Geometry check sheet. Reference: the model listing, model coordinates, mm. A direction names the side the tool comes from. Coordinates: 2 decimals unless noted, no trailing zeros. Order: outer loops, then holes, each group sorted by start corner. A loop starts at its lowest first (then second) coordinate and runs counter-clockwise, first axis right, second up. Notation, with made-up numbers: (36.5, 8.5) - (79.5, 8.5) arc R6 ccw to (79.5, 17.5) - close; hole circle Ø6 at (16.5, 34). An arc over 180 degrees is marked (long way). Return JSON: item names as keys, results as strings. Group by question number.
Item 1: Gauge pin test, flat ends, axial feed: pin 1 (7 mm diameter, centred on x = 54.9, z = 32.5, fed in from -Y); pin 2 (4.5 mm diameter, centred on x = 54.9, z = 92.5, fed in from +Y); pin 3 (8 mm diameter, centred on x = 40.5, y = 24, fed in from -Z). Record the tip position at first contact, or that the pin passes through.
Item 2: Section check B-B on x = 19.9. Enter the section's corners in (y, z), then the cut area to 3 significant figures.
Item 3: Section check A-A on y = 24.9. Enter the section's corners in (x, z), then the cut area to 3 significant figures.
Item 4: Section check D-D on z = 53. Enter the section's corners in (x, y), then the cut area to 3 significant figures.
Item 5: Tool access check on faces 4 (the cylindrical face through (26.908, 28.204, 7.395)), 5 (the cylindrical face through (43.394, 25.164, 69.23)), 6 (the cylindrical face through (60.85, 4.93, 93.28)). Record the directions out of +Z, -Z, +X, -X, +Y, -Y that give a thin tool (end or side, any length) a straight path to the whole face; none if there is none.
Item 6: Scan lines: probe 1 along Z at (x, y) = (54.9, 38); probe 2 along X at (y, z) = (4.25, 92.5); probe 3 along Y at (x, z) = (37.4, 85). Record each from-to range of solid material in increasing order.
Item 7: Draft check along Z on faces 1 (the flat face through (33, 20, 15)), 2 (the flat face through (0, 25, 62)), 3 (the flat face through (52, 10, 31)). Enter one of: pulls with the +Z half, pulls with the -Z half, needs draft (parallel to the pull), parting line crosses it, or undercut.
Item 8: Section check C-C on z = 32.5. Enter the section's corners in (x, y).
from build123d import *

# Parameters (mm, degrees)
SKETCH1_W                        = 74.8
SKETCH1_H                        = 49.8
SLIDER_BODY_DEPTH                = 125
SKETCH2_R                        = 11
LEAD_NUT_INSET_DEPTH             = 15
SKETCH3_R                        = 6
LEADSCREW_CLEARANCE_DEPTH        = 143.039008726
CORNER_BREAK_R                   = 0.5
BOLT_CLEARANCE_HOLES_D           = 5.5
SKETCH7_R                        = 6
NUT_CLEARANCE_COUNTERBORES_DEPTH = 10


with BuildPart() as part:
    # Sketch1 → slider body (new body)
    with BuildSketch(Plane.XY):
        with Locations((37.4, 24.9)):
            Rectangle(SKETCH1_W, SKETCH1_H)
    extrude(amount=SLIDER_BODY_DEPTH)

    # Sketch2 → lead nut inset (cut)
    with BuildSketch(Plane(origin=(0, 0, 0), x_dir=(-1, 0, 0), z_dir=(0, 0, -1))):
        with Locations((-37.4, 24.9)):
            Circle(SKETCH2_R)
    extrude(amount=-LEAD_NUT_INSET_DEPTH, mode=Mode.SUBTRACT)

    # Sketch3 → leadscrew clearance (cut, through all)
    with BuildSketch(Plane(origin=(0, 0, 15), x_dir=(-1, 0, 0), z_dir=(0, 0, -1))):
        with Locations((-37.4, 24.9)):
            Circle(SKETCH3_R)
    extrude(amount=-LEADSCREW_CLEARANCE_DEPTH, mode=Mode.SUBTRACT)

    # corner break
    corner_break_edges = [part.edges().sort_by_distance(p)[0] for p in [
        (74.8, 24.9, 125),
        (37.4, 49.8, 125),
        (0, 24.9, 125),
        (37.4, 49.8, 0),
        (74.8, 24.9, 0),
        (37.4, 0, 0),
        (0, 24.9, 0),
        (37.4, 0, 125),
        (0, 49.8, 62.5),
        (74.8, 49.8, 62.5),
        (74.8, 0, 62.5),
        (0, 0, 62.5),
    ]]
    fillet(corner_break_edges, radius=CORNER_BREAK_R)

    # bolt clearance holes (through all)
    with Locations(Plane(origin=(0, 49.8, 0), x_dir=(1, 0, 0), z_dir=(0, 1, 0))):
        with Locations((54.9, -92.5), (19.9, -32.5), (54.9, -32.5), (19.9, -92.5)):
            Hole(BOLT_CLEARANCE_HOLES_D / 2)

    # Sketch7 → nut clearance counterbores (cut)
    with BuildSketch(Plane.XZ):
        with Locations(Location((19.9, 92.5, 0), (0, 0, 270))):
            Circle(SKETCH7_R)
        with Locations(Location((54.9, 92.5, 0), (0, 0, 270))):
            Circle(SKETCH7_R)
        with Locations(Location((54.9, 32.5, 0), (0, 0, 270))):
            Circle(SKETCH7_R)
        with Locations(Location((19.9, 32.5, 0), (0, 0, 270))):
            Circle(SKETCH7_R)
    extrude(amount=-NUT_CLEARANCE_COUNTERBORES_DEPTH, mode=Mode.SUBTRACT)


solid = part.part
Computed:
{
 "1": {"pin 1": "stops at y = 10", "pin 2": "passes through", "pin 3": "stops at z = 15"},
 "2": {"outline": "(0, 0.5) arc R0.5 ccw to (0.5, 0) - (49.3, 0) arc R0.5 ccw to (49.8, 0.5) - (49.8, 29.75) - (10, 29.75) - (10, 26.5) - (0, 26.5) - close; (0, 38.5) - (10, 38.5) - (10, 35.25) - (49.8, 35.25) - (49.8, 89.75) - (10, 89.75) - (10, 86.5) - (0, 86.5) - close; (0, 98.5) - (10, 98.5) - (10, 95.25) - (49.8, 95.25) - (49.8, 124.5) arc R0.5 ccw to (49.3, 125) - (0.5, 125) arc R0.5 ccw to (0, 124.5) - close", "area": "5,550 mm²"},
 "3": {"outline": "(0, 0.5) arc R0.5 ccw to (0.5, 0) - (26.4, 0) - (26.4, 15) - (31.4, 15) - (31.4, 125) - (0.5, 125) arc R0.5 ccw to (0, 124.5) - close; (43.4, 15) - (48.4, 15) - (48.4, 0) - (74.3, 0) arc R0.5 ccw to (74.8, 0.5) - (74.8, 124.5) arc R0.5 ccw to (74.3, 125) - (43.4, 125) - close; hole circle Ø5.5 at (19.9, 32.5); hole circle Ø5.5 at (19.9, 92.5); hole circle Ø5.5 at (54.9, 32.5); hole circle Ø5.5 at (54.9, 92.5)", "area": "7,600 mm²"},
 "4": {"outline": "(0, 0.5) arc R0.5 ccw to (0.5, 0) - (74.3, 0) arc R0.5 ccw to (74.8, 0.5) - (74.8, 49.3) arc R0.5 ccw to (74.3, 49.8) - (0.5, 49.8) arc R0.5 ccw to (0, 49.3) - close; hole circle Ø12 at (37.4, 24.9)", "area": "3,610 mm²"},
 "5": {"face 4": "-Z", "face 5": "+Z, -Z", "face 6": "-Y"},
 "6": {"probe 1": "z = 0 to 29.75, 35.25 to 89.75, 95.25 to 125", "probe 2": "x = 0 to 13.9, 25.9 to 48.9, 60.9 to 74.8", "probe 3": "y = 0 to 18.9, 30.9 to 49.8"},
 "7": {"face 1": "pulls with the -Z half", "face 2": "needs draft", "face 3": "undercut"},
 "8": {"outline": "(0, 0.5) arc R0.5 ccw to (0.5, 0) - (13.9, 0) - (13.9, 10) - (17.15, 10) - (17.15, 49.8) - (0.5, 49.8) arc R0.5 ccw to (0, 49.3) - close; (22.65, 10) - (25.9, 10) - (25.9, 0) - (48.9, 0) - (48.9, 10) - (52.15, 10) - (52.15, 49.8) - (22.65, 49.8) - close; (57.65, 10) - (60.9, 10) - (60.9, 0) - (74.3, 0) arc R0.5 ccw to (74.8, 0.5) - (74.8, 49.3) arc R0.5 ccw to (74.3, 49.8) - (57.65, 49.8) - close; hole circle Ø12 at (37.4, 24.9)"}
}
